Build history of the part. All positions in model axes, mm. Face numbers are marked on the shaded views. A direction names the side the tool comes from. Give positions to 0.01 mm unless a question says otherwise; leave off trailing zeros. Order: outer loops, then holes, each group sorted by start corner. A loop starts at its lowest first (then second) coordinate and runs counter-clockwise, first axis right, second up. Notation, with made-up numbers: (78.5, 13) -> (101.5, 13) arc R22 ccw to (101.5, 49) -> close; hole circle Ø1 at (48.25, 69.5). An arc over 180 degrees is marked (long way). Write item = value, one per line. Start each with the question number.
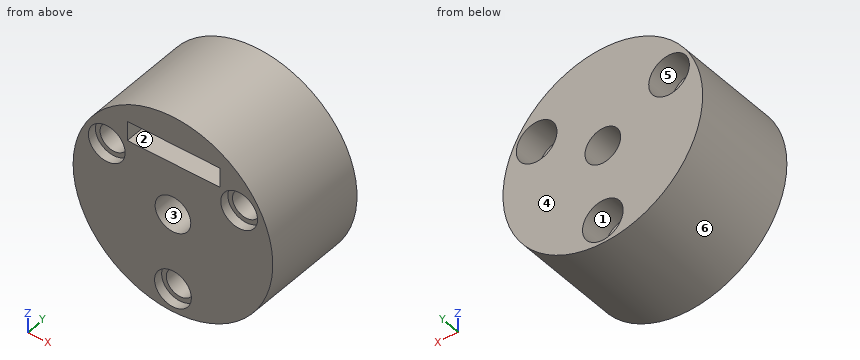
Autodesk Inventor part; units mm, degrees
ref_plane "YZ Plane" through (0, 0, 0) normal (1, 0, 0) x (0, 1, 0)
ref_plane "XZ Plane" through (0, 0, 0) normal (0, 1, 0) x (-1, 0, 0)
ref_plane "XY Plane" through (0, 0, 0) normal (0, 0, 1) x (1, 0, 0)
sketch "Sketch1" plane through (0, 0, 0) normal (0, 1, 0) x (-1, 0, 0)
  line L0 (0, 0) -> (13.6144, 0)
  circle A0 centre (0, 0) radius 17.78
  dimension "d0" = 13.6144
  dimension "d1" = 35.56
extrude "Extrusion1" add sketch "Sketch1" along normal blind 19.05
sketch "Sketch3" plane through (0, 19.05, 0) normal (0, 1, 0) x (1, 0, 0)
  line L0 (0, 0) -> (0, 13.6144)
  line L1 (0, 0) -> (13.6144, 0) construction
  dimension "d4" = 13.6144
  dimension "d5" = 90
hole "Hole1" at (0, 19.05, -13.6144) direction (0, -1, 0) diameter 4.9022 end through all counterbore diameter 7.239 counterbore depth 5.08
sketch "Sketch4" plane through (0, 0, 0) normal (0, -1, 0) x (1, 0, 0)
  circle A0 centre (0, -13.6144) radius 2.4511
  line L0 (0, 0) -> (0, -13.6144)
hole "Hole2" at (0, 0, -13.6144) direction (0, 1, 0) diameter 4.9022 depth 6.35 counterbore diameter 6.5532 counterbore depth 1.6002
pattern_circular "Circular Pattern1" count 3 over 360 about axis through (0, 0, 0) along (0, 1, 0) of "Hole1", "Hole2"
sketch "Sketch6" plane through (0, 19.05, 0) normal (0, 1, 0) x (1, 0, 0)
  point P0 (0, 0)
  point P1 (0, 0)
hole "Hole3" at (0, 19.05, 0) direction (0, -1, 0) diameter 6.35 end through all
sketch "Sketch10" plane through (0, 0, 0) normal (0, -1, 0) x (1, 0, 0)
  circle A0 centre (0, 0) radius 15.24
  circle A1 centre (11.7904, 6.8072) radius 2.4511
  circle A2 centre (-11.7904, 6.8072) radius 2.4511
  line L0 (11.7904, 6.8072) -> (-11.7904, 6.8072)
  line L1 (8.3352, 12.7586) -> (-8.1178, 12.7586)
  line L2 (-8.1178, 12.7586) -> (-8.1178, 9.2583)
  line L3 (-8.1178, 9.2583) -> (8.3352, 9.2583)
  line L4 (8.3352, 9.2583) -> (8.3352, 12.7586)
  dimension "d38" = 30.48
extrude "Extrusion2" cut sketch "Sketch10" against normal blind 5.08 contours L4 L3 L2 L1
properties part number "tablecut"
(1) Flat gauge pins, fed straight in: P1, Ø4, axis at x = 0, z = -13.61, coming from the +Y side; P2, Ø5, axis at x = 0, z = -13.61, coming from the -Y side; P3, Ø10, axis at y = 12.5, z = 12, coming from the -X side; P4, Ø2.5, axis at x = 2.5, y = 2, coming from the +Z side. Where does each tip first touch, or does it go through?
(2) 3-axis set-ups, long thin cutter, end or side, ignore diameter. For the marked faces 1, 2 and 3: which of +Z, -Z, +X, -X, +Y, -Y reach the whole face in a straight line?
(3) Mould opens along X. For the marked faces 4, 5 and 6 say: released by +X, released by -X, zero draft, split by the parting line, or undercut.
(4) Cut at B-B, the plane z = 0. Give the cut face in (x, y) (3 decimals), plus the area to 3 significant figures.
(5) Wall check: line 1 (Z direction, x = 0, y = 15.1) (3 decimals); line 2 (X direction, y = 16, z = 9); line 3 (Z direction, x = -2.5, y = 1.5). Give the ranges that are in metal, low to high. Write a range as [from, to].
(6) Cut at C-C, the plane z = 7. Give the cut face in (x, y), plus the area to 3 significant figures.
(7) Cut at A-A, the plane x = 0. Give the number of separate pieces and of enclosed holes in the cut face, plus the area to 3 significant figures.
(8) Cut at D-D, the plane x = 13. Give the cut face in (y, z), plus the area to 3 significant figures.
Results:
q1.P1 = through
q1.P2 = 1.6
q1.P3 = -16.34
q1.P4 = 17.74
q2.face_1 = +Y
q2.face_2 = -Y
q2.face_3 = +Y, -Y
q3.face_4 = zero draft
q3.face_5 = undercut
q3.face_6 = split by the parting line
q4.outline = (-17.78, 0) -> (-3.175, 0) -> (-3.175, 19.05) -> (-17.78, 19.05) -> close; (3.175, 0) -> (17.78, 0) -> (17.78, 19.05) -> (3.175, 19.05) -> close
q4.area = 556 mm2
q5.line_1 = [-17.78, -17.234], [-9.995, -3.175], [3.175, 17.78]
q5.line_2 = [-15.33, -14.67], [-8.91, 8.91], [14.67, 15.33]
q5.line_3 = [-17.6, -15.73], [-11.5, -1.96], [1.96, 9.26], [12.76, 17.6]
q6.outline = (-16.34, 0) -> (-15.06, 0) -> (-15.06, 1.6) -> (-14.23, 1.6) -> (-14.23, 13.97) -> (-15.4, 13.97) -> (-15.4, 19.05) -> (-16.34, 19.05) -> close; (-9.35, 1.6) -> (-8.52, 1.6) -> (-8.52, 0) -> (8.52, 0) -> (8.52, 1.6) -> (9.35, 1.6) -> (9.35, 13.97) -> (8.18, 13.97) -> (8.18, 19.05) -> (-8.18, 19.05) -> (-8.18, 13.97) -> (-9.35, 13.97) -> close; (14.23, 1.6) -> (15.06, 1.6) -> (15.06, 0) -> (16.34, 0) -> (16.34, 19.05) -> (15.4, 19.05) -> (15.4, 13.97) -> (14.23, 13.97) -> close
q6.area = 407 mm2
q7.separate_pieces = 3
q7.enclosed_holes = 0
q7.area = 431 mm2
q8.outline = (0, -12.13) -> (19.05, -12.13) -> (19.05, 3.4) -> (13.97, 3.4) -> (13.97, 4.68) -> (1.6, 4.68) -> (1.6, 3.76) -> (0, 3.76) -> close; (0, 9.85) -> (1.6, 9.85) -> (1.6, 8.94) -> (13.97, 8.94) -> (13.97, 10.22) -> (19.05, 10.22) -> (19.05, 12.13) -> (0, 12.13) -> close
q8.area = 365 mm2
